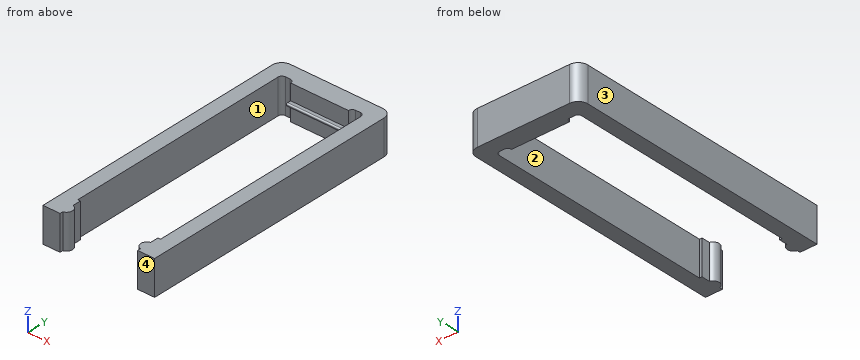
from build123d import *

# Parameters (mm, degrees)
F2_DEPTH = 18
F3_W     = 30
F3_H     = 1.5
F4_DEPTH = 2.5
F5_R     = 0.75
F6_R     = 0.74999


# Not quite as in the source:
# - a fillet or chamfer is up to 0.001 mm smaller than in the source, because OpenCascade refuses the exact size


with BuildPart() as f2:
    # F1 (on Top) → F2 (new body)
    with BuildSketch(Plane.XY):
        with BuildLine():
            Line((24, 140), (0, 140))
            Line((0, 140), (-24, 140))
            ThreePointArc((-24, 140), (-27.5355339059, 138.5355339059), (-29, 135))
            Line((-29, 135), (-29, 0))
            Line((-29, 0), (-20.15, 0))
            Line((-20.15, 0), (-20.15, 1.6))
            ThreePointArc((-20.15, 1.6), (-17.75, 4.65), (-20.15, 7.7))
            Line((-20.15, 7.7), (-20.15, 12))
            Line((-20.15, 12), (-21.5, 12))
            Line((-21.5, 12), (-21.5, 130))
            ThreePointArc((-21.5, 130), (-20.9142135624, 131.4142135624), (-19.5, 132))
            Line((-19.5, 132), (-17, 132))
            ThreePointArc((-17, 132), (-15.5857864376, 131.4142135624), (-15, 130))
            Line((-15, 130), (0, 130))
            Line((0, 130), (15, 130))
            ThreePointArc((15, 130), (15.5857864376, 131.4142135624), (17, 132))
            Line((17, 132), (19.5, 132))
            ThreePointArc((19.5, 132), (20.9142135624, 131.4142135624), (21.5, 130))
            Line((21.5, 130), (21.5, 12))
            Line((21.5, 12), (20.15, 12))
            Line((20.15, 12), (20.15, 7.7))
            ThreePointArc((20.15, 7.7), (17.75, 4.65), (20.15, 1.6))
            Line((20.15, 1.6), (20.15, 0))
            Line((20.15, 0), (29, 0))
            Line((29, 0), (29, 135))
            ThreePointArc((29, 135), (27.5355339059, 138.5355339059), (24, 140))
        make_face()
    extrude(amount=F2_DEPTH)

    # F3 (on face) → F4 (join)
    with BuildSketch(Plane.XZ.offset(-130)):
        with Locations((0, 9)):
            Rectangle(F3_W, F3_H)
    extrude(amount=F4_DEPTH)

    # F5
    f5_edges = [f2.edges().sort_by_distance(p)[0] for p in [
        (0, 127.5, 9.75),
    ]]
    fillet(f5_edges, radius=F5_R)

    # F6 (radius 0.75 in the source; OpenCascade refuses exactly that, so slightly less here)
    f6_edges = [f2.edges().sort_by_distance(p)[0] for p in [
        (0, 127.5, 8.25),
    ]]
    fillet(f6_edges, radius=F6_R)


solid = f2.part
Read the model definition and answer for the solid it produces. Units are mm, in the model's axes. Face numbers are marked on the shaded views. Round coordinates to 2 decimals unless told otherwise and drop trailing zeros. Loops run counter-clockwise (first coordinate to the right, second up) from the corner with the lowest first, then second, coordinate; pieces in that order, holes last.
Q1. Section C-C on z = 16.5 is taken. Write down the section's boundary in (x, y).
Q2. Determine the mould class of the marked faces 1, 2, 3 and 4 for opening direction Y: released by +Y, released by -Y, zero draft, split by the parting line, or undercut.
Q3. Each of these flat-tipped pins is pushed along its axis until it touches: pin 1 (3 mm diameter, centred on x = -21.5, z = 6, fed in from -Y); pin 2 (2 mm diameter, centred on x = 18.5, z = 13.5, fed in from -Y); pin 3 (0.8 mm diameter, centred on x = -18, z = 12, fed in from -Y); pin 4 (9 mm diameter, centred on x = -7, z = 15, fed in from -Y). Where does it stop, or does it pass through?
Q4. Consider probe 1 along X at (y, z) = (109.5, 6); probe 2 along Y at (x, z) = (-13.5, 16); probe 3 along Y at (x, z) = (14, 9). Determine where each line is inside the solid, lowest interval first.
Q5. Section A-A on y = 40.5 is taken. Write down the section's boundary in (x, z).
Output:
1. outline: (-29, 0) - (-20.15, 0) - (-20.15, 1.6) arc R3.14 ccw to (-20.15, 7.7) - (-20.15, 12) - (-21.5, 12) - (-21.5, 130) arc R2 cw to (-19.5, 132) - (-17, 132) arc R2 cw to (-15, 130) - (15, 130) arc R2 cw to (17, 132) - (19.5, 132) arc R2 cw to (21.5, 130) - (21.5, 12) - (20.15, 12) - (20.15, 7.7) arc R3.14 ccw to (20.15, 1.6) - (20.15, 0) - (29, 0) - (29, 135) arc R5 ccw to (24, 140) - (-24, 140) arc R5 ccw to (-29, 135) - close
2. face 1: undercut
2. face 2: undercut
2. face 3: zero draft
2. face 4: released by -Y
3. pin 1: stops at y = 0
3. pin 2: stops at y = 1.84
3. pin 3: stops at y = 2.74
3. pin 4: stops at y = 130
4. probe 1: x = -29 to -21.5, 21.5 to 29
4. probe 2: y = 130 to 140
4. probe 3: y = 127.5 to 140
5. outline: (-29, 0) - (-21.5, 0) - (-21.5, 18) - (-29, 18) - close; (21.5, 0) - (29, 0) - (29, 18) - (21.5, 18) - close
